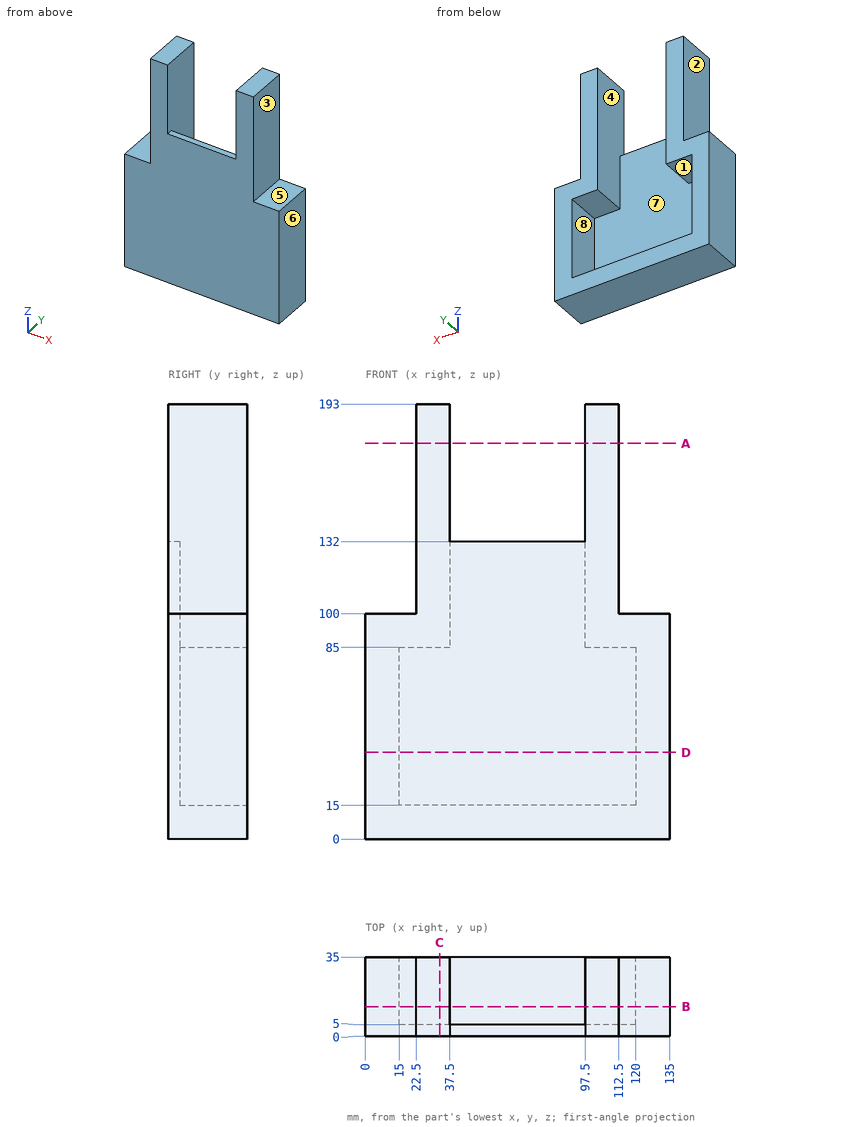
Geometry check sheet. Reference: drawing and pictorial views, mm from the part's lowest x, y, z. A direction names the side the tool comes from. Give positions to 0.01 mm unless a question says otherwise; leave off trailing zeros. Write each loop counter-clockwise with the first axis right and the second up, starting at its lowest first coordinate (ties: lowest second). Pieces come first, ordered by that corner, then holes. Notation, with made-up numbers: (21, 17.5) - (29, 17.5) arc R29 ccw to (29, 38.5) - close; hole circle Ø11 at (1, -4.75). An arc over 180 degrees is marked (long way). Put each result on its own line as item: value.
Q1. Depth check by flat-ended pin: P1, Ø4, axis at x = 79.5, y = 2, coming from the +Z side; P2, Ø6, axis at x = 48.5, z = 50, coming from the +Y side; P3, Ø2, axis at x = 51.5, y = 30, coming from the +Z side. Enter the tip coordinate at first touch or a pass-through.
Result:
P1: z = 132
P2: y = 5
P3: z = 15
Q2. Scan lines: probe 1 along X at (y, z) = (12, 154); probe 2 along Z at (x, y) = (18, 27); probe 3 along X at (y, z) = (21, 76.5). Record each from-to range of solid material in increasing order. Write a range as from..to.
Result:
probe 1: 22.5..37.5, 97.5..112.5
probe 2: 0..15, 85..100
probe 3: 0..15, 120..135
Q3. Set-up check for the marked faces 1, 2, 3 and 4: record each of +Z, -Z, +X, -X, +Y, -Y from which the full face is reachable in a straight line by a thin tool's end or side.
Result:
face 1: +Y
face 2: +Z, -X, +Y, -Y
face 3: +Z, +X, +Y, -Y
face 4: +Z, +Y
Q4. Section check D-D on z = 38.5. Record the cut outline in (x, y), and give its area (4 significant figures).
Result:
outline: (0, 0) - (135, 0) - (135, 35) - (120, 35) - (120, 5) - (15, 5) - (15, 35) - (0, 35) - close
area: 1,575 mm2
Q5. Section check C-C on x = 33. Record the cut outline in (y, z), and give its area (4 significant figures).
Result:
outline: (0, 0) - (35, 0) - (35, 15) - (5, 15) - (5, 85) - (35, 85) - (35, 193) - (0, 193) - close
area: 4,655 mm2
Q6. Section check B-B on y = 13. Record the cut outline in (x, z), and give its area (3 significant figures).
Result:
outline: (0, 0) - (135, 0) - (135, 100) - (112.5, 100) - (112.5, 193) - (97.5, 193) - (97.5, 85) - (120, 85) - (120, 15) - (15, 15) - (15, 85) - (37.5, 85) - (37.5, 193) - (22.5, 193) - (22.5, 100) - (0, 100) - close
area: 8,040 mm2
Q7. Section check A-A on z = 175.5. Record the cut outline in (x, y), and give its area (3 significant figures).
Result:
outline: (22.5, 0) - (37.5, 0) - (37.5, 35) - (22.5, 35) - close; (97.5, 0) - (112.5, 0) - (112.5, 35) - (97.5, 35) - close
area: 1,050 mm2
Q8. Mould release check, pull along Z, two halves, no side actions. Record for the marked faces 5, 6, 7 and 8: released by +Z, released by -Z, zero draft, split by the parting line, or undercut.
Result:
face 5: released by +Z
face 6: zero draft
face 7: undercut
face 8: undercut
